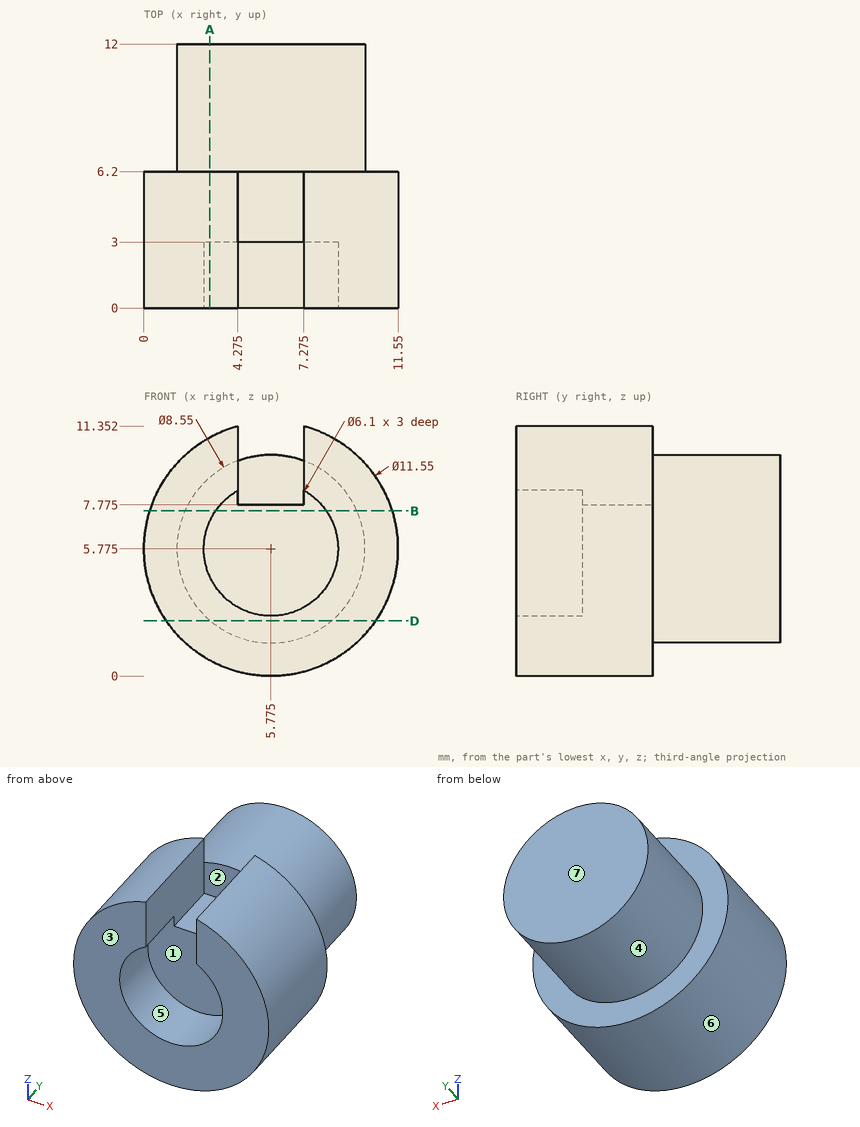
Design review of the part shown in the three views and the two pictorial views. Dimensions are in mm from the part's minimum x, y and z. A direction names the side the tool comes from. Round coordinates to 2 decimals unless told otherwise and drop trailing zeros. Write each loop counter-clockwise with the first axis right and the second up, starting at its lowest first coordinate (ties: lowest second). Pieces come first, ordered by that corner, then holes.
Item 1: We need section D-D on z = 2.5. Write out the cut boundary in (x, y).
Item 2: For the marked faces 1, 2, 3 and 4, list the 3-axis set-ups (+Z, -Z, +X, -X, +Y, -Y) from which the entire face can be reached by the end or side of a thin tool; tool diameter is ignored.
Item 3: Clearance check with flat-ended pins moving along their axes: pin 1 Ø4 at (y, z) = (10, 2) entering from -X; pin 2 Ø1 at (y, z) = (6, 7) entering from +X; pin 3 Ø1.1 at (y, z) = (3.5, 9.5) entering from +X. State where each tip first meets the part, or that it passes through.
Item 4: We need section A-A on x = 3. Write out the cut boundary in (y, z).
Item 5: The part is to be moulded in two halves that separate along X. For the marked faces 5, 6 and 7, say which applies: +X half, -X half, draft (parallel to the pull), parting line (faces both ways), or undercut.
Item 6: For probe 1 along Y at (x, z) = (5.5, 3.5); probe 2 along X at (y, z) = (5.75, 9.5) (1 decimal); probe 3 along Y at (x, z) = (8.25, 10.5), list the stretches that pass through material, from the lowest coordinate up.
Item 7: We need section B-B on z = 7.5. Write out the cut boundary in (x, y).
Returned:
1. outline: (1.02, 0) - (10.53, 0) - (10.53, 6.2) - (8.52, 6.2) - (8.52, 12) - (3.03, 12) - (3.03, 6.2) - (1.02, 6.2) - close
2. face 1: -Y
2. face 2: +Z, -Y
2. face 3: +Z, -Z, +X, -X, -Y
2. face 4: +Y
3. pin 1: stops at x = 1.89
3. pin 2: stops at x = 11.5
3. pin 3: stops at x = 10.6
4. outline: (0, 0.71) - (6.2, 0.71) - (6.2, 2.52) - (12, 2.52) - (12, 9.03) - (6.2, 9.03) - (6.2, 10.84) - (0, 10.84) - (0, 7.04) - (3, 7.04) - (3, 4.51) - (0, 4.51) - close
5. face 5: undercut
5. face 6: parting line
5. face 7: draft
6. probe 1: y = 3 to 12
6. probe 2: x = 1.4 to 4.3, 7.3 to 10.2
6. probe 3: y = 0 to 6.2
7. outline: (0.26, 0) - (3.26, 0) - (3.26, 3) - (8.29, 3) - (8.29, 0) - (11.29, 0) - (11.29, 6.2) - (9.69, 6.2) - (9.69, 12) - (1.86, 12) - (1.86, 6.2) - (0.26, 6.2) - close
